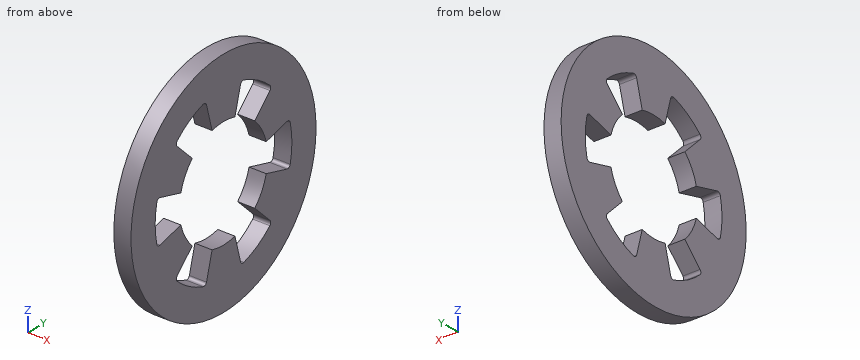
Autodesk Inventor part; units mm, degrees
ref_plane "Work Plane1" through (0, 0, 0) normal (0, 1, 0) x (1, 0, 0)
ref_plane "YZ Plane" through (0, 0, 0) normal (1, 0, 0) x (0, 1, 0)
ref_plane "XZ Plane" through (0, 0, 0) normal (0, 1, 0) x (-1, 0, 0)
sketch "Sketch1" plane through (0, 0, 0) normal (1, 0, 0) x (0, 1, 0)
  circle A0 centre (0, 0) radius 3.7465
  circle A1 centre (0, 0) radius 1.7907
  dimension "d0" = 7.493
  dimension "d1" = 3.5814
extrude "Body" add sketch "Sketch1" along normal blind 0.5588
sketch "Sketch2" plane through (0, 0, 0) normal (-1, 0, 0) x (0, 0, 1)
  circle A0 centre (0, 0) radius 1.7907
  circle A1 centre (0, 0) radius 3.7465
  arc A2 (0.7166, 2.6743) -> (-0.7166, 2.6743) centre (0, 0) ccw
  line L0 (-0.4635, 1.7297) -> (-0.7166, 2.6743)
  line L1 (0, 0) -> (0, 2.7686) construction
  line L2 (0.4635, 1.7297) -> (0.7166, 2.6743)
  line L3 (-0.4635, 1.7297) -> (0, 0) construction
  line L4 (0.4635, 1.7297) -> (0, 0) construction
  dimension "d4" = 5.5372
  dimension "d5" = 15
extrude "Cut" cut sketch "Sketch2" against normal blind 0.5588 contours A0 L0 A2 L2
fillet "Fillet1" radius 0.1074 2 edges at (0.2794, 2.6743, 0.7166) (0.2794, 2.6743, -0.7166)
pattern_circular "Cuts" count 6 over 360 about axis through (-10, 0, 0) along (1, 0, 0) of "Cut", "Fillet1"
ref_plane "Work Plane1" through (0, 0, 0) normal (0, 1, 0) x (1, 0, 0)
equation "\"d0\" = SD2"
equation "\"d1\" = SD1"
equation "\"d2\" = SD"
equation "\"d4\" = 0.5 * SD2 + 0.5 * SD1"
equation "\"d6\" = SD"
equation "\"d8\" = 0.03 * SD1"
equation "\"SD1\" = 3.5814"
equation "\"SD2\" = 7.493"
equation "\"SD\" = 0.5588"
equation "\"NND\" = 3.5052"
properties part number "ASME B18.21.1 - No. 6. Carbon Steel" material "Steel, Mild"
Read the model definition and answer for the solid it produces. Units are mm, in the model's axes. Coordinates: 2 decimals unless noted, no trailing zeros. Loops run counter-clockwise (first coordinate to the right, second up) from the corner with the lowest first, then second, coordinate; pieces in that order, holes last. Notation, with made-up numbers: (68.25, 31.25) -> (79.25, 31.25) arc R28 ccw to (79.25, 51.25) -> close; hole circle Ø6 at (-17.75, 16.25). An arc over 180 degrees is marked (long way). Return JSON: item names as keys, results as strings.
Item 1: Find section D-D (y = -3). Determine the outline of the cut face in (x, z).
Answers:
{"outline": "(0, -2.24) -> (0.56, -2.24) -> (0.56, 2.24) -> (0, 2.24) -> close"}
Item 2: Find section C-C (z = 2.25). Determine the outline of the cut face in (x, y), plus the area to 3 significant figures.
Answers:
{"outline": "(0, -3) -> (0.56, -3) -> (0.56, -1.61) -> (0, -1.61) -> close; (0, -0.6) -> (0.56, -0.6) -> (0.56, 0.6) -> (0, 0.6) -> close; (0, 1.61) -> (0.56, 1.61) -> (0.56, 3) -> (0, 3) -> close", "area": "2.22 mm2"}
Item 3: Find the intervals of material crossed by probe 1 along Z at (x, y) = (0.35, -1.5); probe 2 along Z at (x, y) = (0.2, -2); probe 3 along Y at (x, z) = (0.5, 0.25), in increasing order.
Answers:
{"probe 1": "z = -3.43 to -2.33, -1.5 to -0.98, 0.98 to 1.5, 2.33 to 3.43", "probe 2": "z = -3.17 to -0.54, 0.54 to 3.17", "probe 3": "y = -3.74 to -2.76, 2.76 to 3.74"}
Item 4: Find section B-B (z = 0). Determine the outline of the cut face in (x, y), plus the area to 3 significant figures.
Answers:
{"outline": "(0, -3.75) -> (0.56, -3.75) -> (0.56, -2.77) -> (0, -2.77) -> close; (0, 2.77) -> (0.56, 2.77) -> (0.56, 3.75) -> (0, 3.75) -> close", "area": "1.09 mm2"}
Item 5: Find section A-A (y = 0). Determine the outline of the cut face in (x, z).
Answers:
{"outline": "(0, -3.75) -> (0.56, -3.75) -> (0.56, -1.79) -> (0, -1.79) -> close; (0, 1.79) -> (0.56, 1.79) -> (0.56, 3.75) -> (0, 3.75) -> close"}
